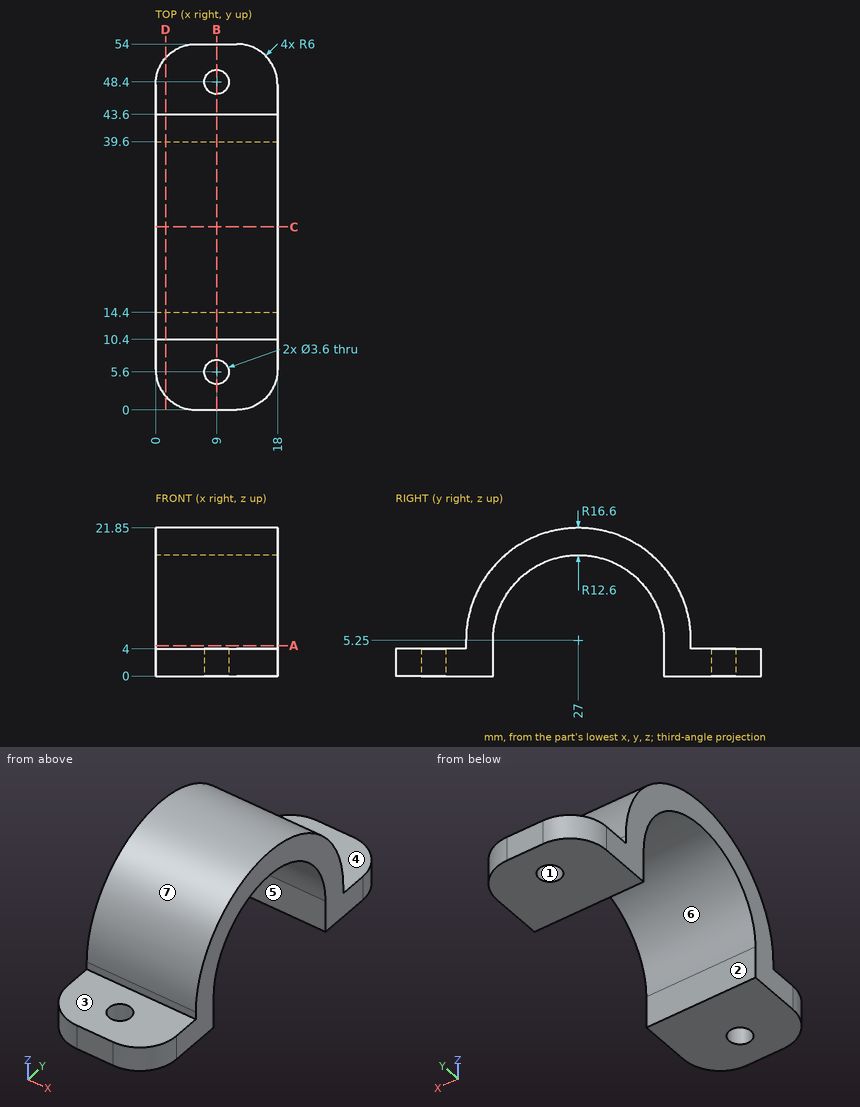
Can you work these out from the drawing? Everything is in mm from the part's minimum corner. A direction names the side the tool comes from. Round coordinates to 2 decimals unless told otherwise and drop trailing zeros. Loops run counter-clockwise (first coordinate to the right, second up) from the corner with the lowest first, then second, coordinate; pieces in that order, holes last. Notation, with made-up numbers: (-17, 46) -> (39, 46) arc R16 cw to (39, 50) -> close; hole circle Ø6 at (-18.5, 18). An arc over 180 degrees is marked (long way). Answer in a Markdown table with one row per item.
Item 1: We'd pull the mould along Y, two halves only. Please class the marked faces 4, 5, 6 and 7: released by +Y, released by -Y, zero draft, split by the parting line, or undercut.
Answer block:
| item | result |
|---|---|
| face 4 | zero draft |
| face 5 | undercut |
| face 6 | undercut |
| face 7 | split by the parting line |
Item 2: If I drill on probe 1 along Y at (x, z) = (9, 1); probe 2 along Z at (x, y) = (13.25, 50.5); probe 3 along Y at (x, z) = (2, 8), over which ranges is the centre line in solid material (lowest first)?
Answer block:
| item | result |
|---|---|
| probe 1 | 0 to 3.8, 7.4 to 14.4, 39.6 to 46.6, 50.2 to 54 |
| probe 2 | 0 to 4 |
| probe 3 | 10.63 to 14.7, 39.3 to 43.37 |
Item 3: Suppose I cut it at C-C, the plane y = 27. List the corners of the cut face in (x, z) for me.
Answer block:
| item | result |
|---|---|
| outline | (0, 17.85) -> (18, 17.85) -> (18, 21.85) -> (0, 21.85) -> close |
Item 4: Suppose I cut it at A-A, the plane z = 4.5. List the corners of the cut face in (x, y) for me.
Answer block:
| item | result |
|---|---|
| outline | (0, 10.4) -> (18, 10.4) -> (18, 14.4) -> (0, 14.4) -> close; (0, 39.6) -> (18, 39.6) -> (18, 43.6) -> (0, 43.6) -> close |
Item 5: Suppose I cut it at D-D, the plane x = 1.5. List the corners of the cut face in (y, z) for me.
Answer block:
| item | result |
|---|---|
| outline | (2.03, 0) -> (14.4, 0) -> (14.4, 5.25) arc R12.6 cw to (39.6, 5.25) -> (39.6, 0) -> (51.97, 0) -> (51.97, 4) -> (43.6, 4) -> (43.6, 5.25) arc R16.6 ccw to (10.4, 5.25) -> (10.4, 4) -> (2.03, 4) -> close |
Item 6: On a 3-axis mill with a long thin cutter (end or side, diameter ignored), from which of +Z, -Z, +X, -X, +Y, -Y can I reach the whole of each face in a straight line? I mean the marked faces 1, 2 and 3. Say none if no direction works.
Answer block:
| item | result |
|---|---|
| face 1 | +Z, -Z |
| face 2 | -Z, +X, -X |
| face 3 | +Z, +X, -X, -Y |
Item 7: Will these pins go through, and if not, where does the flat tip stop? P1, Ø5, axis at x = 8, y = 50.5, coming from the +Z side; P2, Ø1, axis at x = 2, z = 18, coming from the -Y side; P3, Ø4, axis at x = 7, z = 17.5, coming from the -Y side; P4, Ø3, axis at x = 9, y = 48.4, coming from the -Z side.
Answer block:
| item | result |
|---|---|
| P1 | z = 4 |
| P2 | y = 15.8 |
| P3 | y = 13.94 |
| P4 | through |
Item 8: Suppose I cut it at B-B, the plane x = 9. List the corners of the cut face in (y, z) for me, plus the area to 3 significant figures.
Answer block:
| item | result |
|---|---|
| outline | (0, 0) -> (3.8, 0) -> (3.8, 4) -> (0, 4) -> close; (7.4, 0) -> (14.4, 0) -> (14.4, 5.25) arc R12.6 cw to (39.6, 5.25) -> (39.6, 0) -> (46.6, 0) -> (46.6, 4) -> (43.6, 4) -> (43.6, 5.25) arc R16.6 ccw to (10.4, 5.25) -> (10.4, 4) -> (7.4, 4) -> close; (50.2, 0) -> (54, 0) -> (54, 4) -> (50.2, 4) -> close |
| area | 280 mm² |
